CAD build for the part. Positions are in the model's coordinates, mm. A direction names the side the tool comes from. Give positions to 0.01 mm unless a question says otherwise; leave off trailing zeros. Order: outer loops, then holes, each group sorted by start corner. A loop starts at its lowest first (then second) coordinate and runs counter-clockwise, first axis right, second up. Notation, with made-up numbers: (1.5, 38.5) -> (25.5, 38.5) arc R17 cw to (25.5, 62.5) -> close; hole circle Ø2 at (88, 61). An arc over 180 degrees is marked (long way). Use one line per item in the form item = value. Start each with the question number.
1) Drop flat-ended pins along their axis: P1, Ø2, axis at y = 9.5, z = 3.5, coming from the +X side; P2, Ø6, axis at x = 5.5, z = 6, coming from the +Y side. Give the stop position or say it passes through.
2) Cut at A-A, the plane z = 5. Give the cut face in (x, y), and give its area (3 significant figures).
3) Cut at C-C, the plane y = 9.5. Give the cut face in (x, z).
4) Cut at D-D, the plane z = 1.25. Give the cut face in (x, y).
5) Cut at B-B, the plane x = 5. Give the cut face in (y, z), and give its area (3 significant figures).
6) Tool access for faces 1 (the face through (10, 1, 5)), 2 (the face through (0, 15.3, 7.3)), 3 (the face through (-1, 4, 5)): list every direction of +Z, -Z, +X, -X, +Y, -Y with a clear straight run to the whole face (end or side of a thin tool).
7) Probe line 1 (Z direction, x = 5, y = 1.3); line 2 (X direction, y = 0.85, z = 5); line 3 (Y direction, x = 6.75, z = 8). List the from-to ranges inside material, lowest first.
8) Mould opens along Z. For faces 4 (the face through (-1, 15, 7)), 5 (the face through (-0.4, 11, 10)), 6 (the face through (-1, 16, 3)), 7 (the face through (3.8, 3, 3.8)) say: pulls with the +Z half, pulls with the -Z half, needs draft (parallel to the pull), parting line crosses it, or undercut.
from build123d import *

# Parameters (mm, degrees)
SKETCH_2_W          = 10
SKETCH_2_H          = 10
EXTRUDE_2_DEPTH     = 3
SKETCH_3_R          = 1.5
CUT_EXTRUDE_1_DEPTH = 3
EXTRUDE_3_DEPTH     = 10
CUT_EXTRUDE_2_DEPTH = 10


with BuildPart() as part:
    # 草图2 → 凸台-拉伸2 (new body)
    with BuildSketch(Plane(origin=(0, 0, 0), x_dir=(1, 0, 0), z_dir=(0, 1, 0))):
        with Locations((5, -5)):
            Rectangle(SKETCH_2_W, SKETCH_2_H)
    extrude(amount=EXTRUDE_2_DEPTH)

    # 草图3 → 切除-拉伸1 (cut)
    with BuildSketch(Plane(origin=(0, 3, 0), x_dir=(1, 0, 0), z_dir=(0, 1, 0))):
        with Locations((5, -5)):
            Circle(SKETCH_3_R)
    extrude(amount=-CUT_EXTRUDE_1_DEPTH, mode=Mode.SUBTRACT)

    # 草图5 → 凸台-拉伸3 (add, through all)
    with BuildSketch(Plane.XY.offset(10)):
        Polygon((0, 3), (0, 28), (-3, 28), (-3, 0), (0, 0), align=None)
    extrude(amount=-EXTRUDE_3_DEPTH)

    # 草图6 → 切除-拉伸2 (cut)
    with BuildSketch(Plane(origin=(0, 0, 0), x_dir=(0, 0, -1), z_dir=(1, 0, 0))):
        with BuildLine():
            Line((-3, 25), (-3, 6))
            ThreePointArc((-3, 6), (-5, 4), (-7, 6))
            Line((-7, 6), (-7, 25))
            ThreePointArc((-7, 25), (-5, 27), (-3, 25))
        make_face()
    extrude(amount=-CUT_EXTRUDE_2_DEPTH, mode=Mode.SUBTRACT)


solid = part.part
Result:
q1.P1 = 0
q1.P2 = 3
q2.outline = (-3, 0) -> (3.5, 0) -> (3.5, 3) -> (0, 3) -> (0, 4) -> (-3, 4) -> close; (-3, 27) -> (0, 27) -> (0, 28) -> (-3, 28) -> close; (6.5, 0) -> (10, 0) -> (10, 3) -> (6.5, 3) -> close
q2.area = 36.0 mm²
q3.outline = (-3, 0) -> (0, 0) -> (0, 3) -> (-3, 3) -> close; (-3, 7) -> (0, 7) -> (0, 10) -> (-3, 10) -> close
q4.outline = (-3, 0) -> (10, 0) -> (10, 3) -> (0, 3) -> (0, 28) -> (-3, 28) -> close
q5.outline = (0, 0) -> (3, 0) -> (3, 3.5) -> (0, 3.5) -> close; (0, 6.5) -> (3, 6.5) -> (3, 10) -> (0, 10) -> close
q5.area = 21.0 mm²
q6.face_1 = +Z, -Z, +X, +Y, -Y
q6.face_2 = +Z, -Z, +X, +Y
q6.face_3 = +X, -X
q7.line_1 = 0 to 3.5, 6.5 to 10
q7.line_2 = -3 to 3.5, 6.5 to 10
q7.line_3 = 0 to 3
q8.face_4 = undercut
q8.face_5 = pulls with the +Z half
q8.face_6 = undercut
q8.face_7 = needs draft
